from build123d import *

# Parameters (mm, degrees)
SKETCH1_R           = 2
BOSS_EXTRUDE1_DEPTH = 130


with BuildPart() as part:
    # Sketch1 → Boss-Extrude1 (new body, symmetric)
    with BuildSketch(Plane.XY):
        Polygon((10, 10), (10, 4.610379336), (8.2, 3.1), (8.2, 5.5), (6.560660172, 5.5), (3.9, 2.839339828), (3.9, 0.519615242), (3.6, 0), (3.9, -0.519615242), (3.9, -2.839339828), (6.560660172, -5.5), (8.2, -5.5), (8.2, -3.1), (10, -4.610379336), (10, -10), (4.610379336, -10), (3.1, -8.2), (5.5, -8.2), (5.5, -6.560660172), (2.839339828, -3.9), (0.519615242, -3.9), (0, -3.6), (-0.519615242, -3.9), (-2.839339828, -3.9), (-5.5, -6.560660172), (-5.5, -8.2), (-3.1, -8.2), (-4.610379336, -10), (-10, -10), (-10, -4.610379336), (-8.2, -3.1), (-8.2, -5.5), (-6.560660172, -5.5), (-3.9, -2.839339828), (-3.9, -0.519615242), (-3.6, 0), (-3.9, 0.519615242), (-3.9, 2.839339828), (-6.560660172, 5.5), (-8.2, 5.5), (-8.2, 3.1), (-10, 4.610379336), (-10, 10), (-4.610379336, 10), (-3.1, 8.2), (-5.5, 8.2), (-5.5, 6.560660172), (-2.839339828, 3.9), (-0.519615242, 3.9), (0, 3.6), (0.519615242, 3.9), (2.839339828, 3.9), (5.5, 6.560660172), (5.5, 8.2), (3.1, 8.2), (4.610379336, 10), align=None)
        Circle(SKETCH1_R, mode=Mode.SUBTRACT)
    extrude(amount=BOSS_EXTRUDE1_DEPTH, both=True)


solid = part.part
Could you check a few things on this model? Use its own coordinates, in mm. Round coordinates to 2 decimals unless told otherwise and drop trailing zeros. Write item = value, one per line.
1) I'm going to push flat-ended pins straight in: P1, Ø1.5, axis at x = 1, z = -50, coming from the +Y side; P2, Ø3, axis at x = 2, z = 31, coming from the +Y side; P3, Ø1.2, axis at x = -1, z = 50, coming from the -Y side. Where does each tip first touch, or does it pass through?
Computed:
P1 = 3.9
P2 = 8.68
P3 = -3.9
2) If we mould it in two halves opening along Y, with no side actions, what happens to faces 1 (the flat face through (-10, -7, 2)), 2 (the flat face through (7, 10, 2)), 3 (the cylindrical face through (0, -2, -2))? For each: pulls with the +Y half, pulls with the -Y half, needs draft (parallel to the pull), parting line crosses it, or undercut.
Computed:
face_1 = needs draft
face_2 = pulls with the +Y half
face_3 = undercut
3) I need wall thicknesses on line 1 along X through (y, z) = (-8, -95.5); line 2 along Y through (x, z) = (0, -29). Which ranges of each line are inside material? Lowest first, please. Write a range as from..to.
Computed:
line_1 = -10..-5.5, 5.5..10
line_2 = -3.6..-2, 2..3.6
